For this review, take the finished solid that the model builds, in its own axes (mm). Face numbers are marked on the shaded views. Give positions to 0.01 mm unless a question says otherwise; leave off trailing zeros. Loops run counter-clockwise (first coordinate to the right, second up) from the corner with the lowest first, then second, coordinate; pieces in that order, holes last. Notation, with made-up numbers: (25.25, -2.5) -> (70.25, -2.5) arc R21 ccw to (70.25, 18.5) -> close; hole circle Ø4 at (-12, 15.25). An arc over 180 degrees is marked (long way). One line per question, with ' | ' between items. Start each with the question number.
(1) Insertion check: P1, Ø5, axis at x = 1.5, z = -6.5, coming from the +Y side. The pin has a flat end and moves straight along its axis. Give the tip position at first contact, or say it passes through.
(2) Wall thickness on probe 1 along Z at (x, y) = (54.5, -2.75); probe 2 along X at (y, z) = (-3.25, 46.5); probe 3 along X at (y, z) = (-8.25, 4): over which ranges is each line inside the solid? List them lowest first.
(3) Consider section A-A (y = -8). Write out the cut boundary in (x, z).
(4) Consider section B-B (x = -16). Write out the cut boundary in (y, z), and give its area (3 significant figures).
(5) Draft analysis for pull direction X (two halves, no side actions). For the marked faces 1 and 2, state which applies: +X half, -X half, draft (parallel to the pull), parting line (faces both ways), or undercut.
(6) Consider section C-C (z = 30.5). Write out the cut boundary in (x, y), and give its area (3 significant figures).
from build123d import *

# Parameters (mm, degrees)
F0_W     = 129.422773
F0_H     = 103.397541
F1_DEPTH = 10.414
F2_T     = -2.54
F3_W     = 115.706771
F3_H     = 90.560776
F4_DEPTH = 1.27


with BuildPart() as f1:
    # F0 (on Front) → F1 (new body)
    with BuildSketch(Plane.XZ):
        with Locations((-2.286001, 2.637691)):
            Rectangle(F0_W, F0_H)
    extrude(amount=F1_DEPTH)

    # F2
    f2_openings = [f1.faces().sort_by_distance(p)[0] for p in [
        (-2.286, -10.414, 2.637692),
    ]]
    offset(amount=F2_T, openings=f2_openings)

    # F3 (on face) → F4 (join)
    with BuildSketch(Plane.XZ.offset(2.54)):
        with Locations((-2.285999, 2.198076)):
            Rectangle(F3_W, F3_H)
    extrude(amount=F4_DEPTH)


solid = f1.part
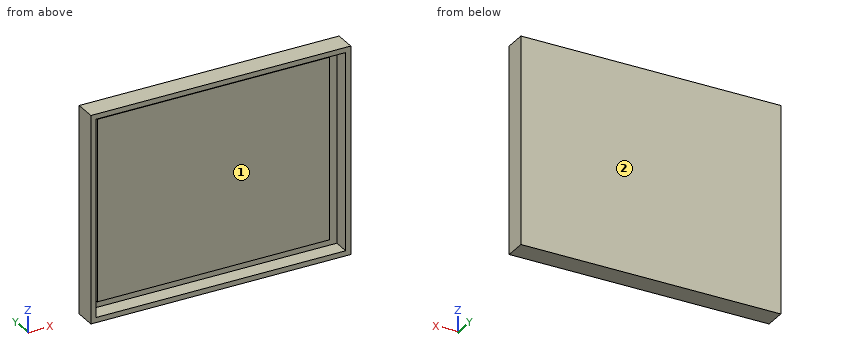
A:
1) P1: stops at y = 0
2) probe 1: z = -49.06 to -46.52, -43.08 to 47.48, 51.8 to 54.34 | probe 2: x = -67 to -64.46, -60.14 to 55.57, 59.89 to 62.43 | probe 3: x = -67 to -64.46, 59.89 to 62.43
3) outline: (-67, -49.06) -> (62.43, -49.06) -> (62.43, 54.34) -> (-67, 54.34) -> close; hole (-64.46, -46.52) -> (59.89, -46.52) -> (59.89, 51.8) -> (-64.46, 51.8) -> close
4) outline: (-10.41, -49.06) -> (0, -49.06) -> (0, 54.34) -> (-10.41, 54.34) -> (-10.41, 51.8) -> (-2.54, 51.8) -> (-2.54, 47.48) -> (-3.81, 47.48) -> (-3.81, -43.08) -> (-2.54, -43.08) -> (-2.54, -46.52) -> (-10.41, -46.52) -> close | area: 418 mm^2
5) face 1: undercut | face 2: draft
6) outline: (-67, -10.41) -> (-64.46, -10.41) -> (-64.46, -2.54) -> (-60.14, -2.54) -> (-60.14, -3.81) -> (55.57, -3.81) -> (55.57, -2.54) -> (59.89, -2.54) -> (59.89, -10.41) -> (62.43, -10.41) -> (62.43, 0) -> (-67, 0) -> close | area: 516 mm^2
